Design review of the part built by this model. Coordinates are the model's own, in mm. Face numbers are marked on the shaded views. Coordinates: 2 decimals unless noted, no trailing zeros. Use a Markdown table: item, result. Add a question column.
Q1. Draft analysis for pull direction X (two halves, no side actions). For the marked faces 1 and 2, state which applies: pulls with the +X half, pulls with the -X half, needs draft (parallel to the pull), parting line crosses it, or undercut.
Q2. Clearance check with flat-ended pins moving along their axes: pin 1 Ø2 at (x, z) = (-7.5, 1371) entering from -Y; pin 2 Ø8 at (y, z) = (594, 1359.5) entering from +X; pin 3 Ø2 at (x, z) = (-17, 1375) entering from +Y. State where each tip first meets the part, or that it passes through.
Q3. For probe 1 along Y at (x, z) = (2, 1361); probe 2 along X at (y, z) = (564.5, 1351); probe 3 along X at (y, z) = (576, 1373.5), list the stretches that pass through material, from the lowest coordinate up.
Q4. Take a section at A-A on z = 1381. Count the separate pieces of the cut face and the enclosed holes in it, plus the area to 3 significant figures.
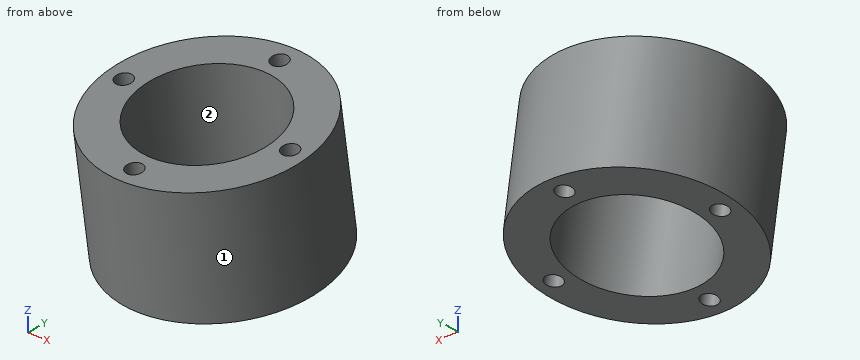
from build123d import *

# Parameters (mm, degrees)
SKETCH1_R                   = 31.75
SKETCH1_R_2                 = 20.6375
BOSS_EXTRUDE1_DEPTH         = 19.05
F_1_4_20_TAPPED_HOLE1_D     = 5.1054
F_1_4_20_TAPPED_HOLE1_DEPTH = 38.1


with BuildPart() as part:
    # Sketch1 → Boss-Extrude1 (new body, symmetric)
    with BuildSketch(Plane(origin=(0, 577.92693102, 1367.654430732), x_dir=(0.999987453, -0.000687148, 0.004962002), z_dir=(-0.005009211, -0.144685018, 0.989465084))):
        Circle(SKETCH1_R)
        Circle(SKETCH1_R_2, mode=Mode.SUBTRACT)
    extrude(amount=BOSS_EXTRUDE1_DEPTH, both=True)

    # 1/4-20 Tapped Hole1
    with Locations(Plane(origin=(-6.264413672, -180.940036548, 1237.404194636), x_dir=(-0.999987401, 0.001044934, -0.004909685), z_dir=(0.005009211, 0.144685018, -0.989465084))):
        with Locations((-32.304604681, 769.73877208), (-6.101384965, 795.923048939), (20.082891894, 769.719829223), (-6.120327822, 743.535552364)):
            Hole(F_1_4_20_TAPPED_HOLE1_D / 2, depth=F_1_4_20_TAPPED_HOLE1_DEPTH)


solid = part.part
Answer list:
| question | item | result |
|---|---|---|
| 1 | face 1 | parting line crosses it |
| 1 | face 2 | undercut |
| 2 | pin 1 | y = 545.98 |
| 2 | pin 2 | x = 29.94 |
| 2 | pin 3 | y = 604.6 |
| 3 | probe 1 | 546.88 to 550.81, 554.05 to 558.14, 599.66 to 603.71, 607.04 to 610.93 |
| 3 | probe 2 | -27.53 to -13.33, 13.47 to 27.67 |
| 3 | probe 3 | -31.76 to -28.55, -23.9 to -20.64, 20.58 to 23.84, 28.49 to 31.7 |
| 4 | separate pieces | 1 |
| 4 | enclosed holes | 5 |
| 4 | area | 1,770 mm² |
